Read the model definition and answer for the solid it produces. Units are mm, in the model's axes. Face numbers are marked on the shaded views. A direction names the side the tool comes from. Give positions to 0.01 mm unless a question says otherwise; leave off trailing zeros. Write each loop counter-clockwise with the first axis right and the second up, starting at its lowest first coordinate (ties: lowest second). Pieces come first, ordered by that corner, then holes. Notation, with made-up numbers: M -27,65 L 16,65 A18 ccw 16,86 Z; hole C -37.5,60 d5. An arc over 180 degrees is marked long. Write each question's results on one line, items separated by ' | '. Start each with the question number.
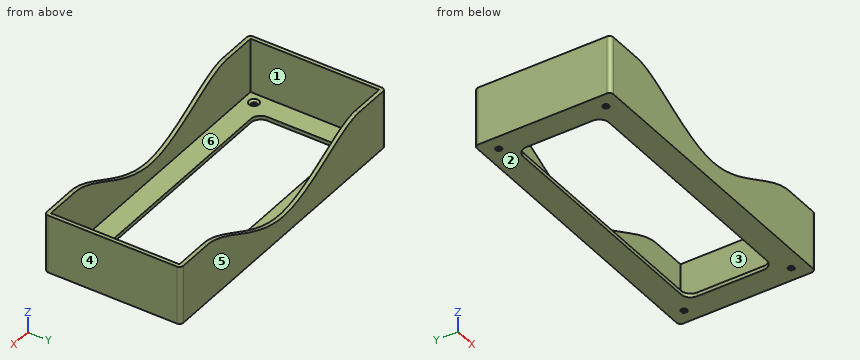
```python
from build123d import *

# Parameters (mm, degrees)
F1_W          = 152
F1_H          = 66
F2_DEPTH      = 30
F1_R          = 1.5875
F3_DEPTH      = 2
F4_SIZE       = 1
F6_DEPTH      = 35
F6_DEPTH_BACK = 35


with BuildPart() as f2:
    # F1 (on Top) → F2 (new body)
    with BuildSketch(Plane.XY):
        with BuildLine():
            ThreePointArc((78, 33), (77.4142135624, 34.4142135624), (76, 35))
            Line((76, 35), (-76, 35))
            ThreePointArc((-76, 35), (-77.4142135624, 34.4142135624), (-78, 33))
            Line((-78, 33), (-78, -33))
            ThreePointArc((-78, -33), (-77.4142135624, -34.4142135624), (-76, -35))
            Line((-76, -35), (76, -35))
            ThreePointArc((76, -35), (77.4142135624, -34.4142135624), (78, -33))
            Line((78, -33), (78, 33))
        make_face()
        Rectangle(F1_W, F1_H, mode=Mode.SUBTRACT)
    extrude(amount=F2_DEPTH)

    # F1 (on Top) → F3 (join)
    with BuildSketch(Plane.XY):
        with BuildLine():
            ThreePointArc((78, 33), (77.4142135624, 34.4142135624), (76, 35))
            Line((76, 35), (-76, 35))
            ThreePointArc((-76, 35), (-77.4142135624, 34.4142135624), (-78, 33))
            Line((-78, 33), (-78, -33))
            ThreePointArc((-78, -33), (-77.4142135624, -34.4142135624), (-76, -35))
            Line((-76, -35), (76, -35))
            ThreePointArc((76, -35), (77.4142135624, -34.4142135624), (78, -33))
            Line((78, -33), (78, 33))
        make_face()
        Rectangle(F1_W, F1_H, mode=Mode.SUBTRACT)
        Rectangle(F1_W, F1_H)
        with Locations((-70.5, -27.5)):
            Circle(F1_R, mode=Mode.SUBTRACT)
        with Locations((70.5, -27.5)):
            Circle(F1_R, mode=Mode.SUBTRACT)
        with Locations((-70.5, 27.5)):
            Circle(F1_R, mode=Mode.SUBTRACT)
        with BuildLine():
            Line((-60, 22), (60, 22))
            ThreePointArc((60, 22), (63.5355339059, 20.5355339059), (65, 17))
            Line((65, 17), (65, -17))
            ThreePointArc((65, -17), (63.5355339059, -20.5355339059), (60, -22))
            Line((60, -22), (-60, -22))
            ThreePointArc((-60, -22), (-63.5355339059, -20.5355339059), (-65, -17))
            Line((-65, -17), (-65, 17))
            ThreePointArc((-65, 17), (-63.5355339059, 20.5355339059), (-60, 22))
        make_face(mode=Mode.SUBTRACT)
        with Locations((70.5, 27.5)):
            Circle(F1_R, mode=Mode.SUBTRACT)
    extrude(amount=F3_DEPTH)

    # F4
    f4_edges = [f2.edges().sort_by_distance(p)[0] for p in [
        (-72.0875, 27.5, 2),
        (68.9125, 27.5, 2),
        (68.9125, -27.5, 2),
        (-72.0875, -27.5, 2),
    ]]
    chamfer(f4_edges, length=F4_SIZE)

    # F5 (on Front) → F6 (cut, two sides)
    with BuildSketch(Plane.XZ) as f6_sk:
        with BuildLine():
            add(Edge.make_bspline(
                [(-58, 30), (-43, 30), (0, -10), (43, 30), (58, 30)],
                knots=[0, 0, 0, 0, 0.5, 1, 1, 1, 1], degree=3))
            Line((58, 30), (-58, 30))
        make_face()
    extrude(amount=-F6_DEPTH, mode=Mode.SUBTRACT)
    extrude(f6_sk.sketch, amount=F6_DEPTH_BACK, mode=Mode.SUBTRACT)


solid = f2.part
```
Item 1: Section B-B, the plane y = 10 is taken. Determine the outline of the cut face in (x, z), then the cut area to 3 significant figures.
Item 2: Straight lines are drawn through the part: line 1 (Y direction, x = -70.5, z = 0.2); line 2 (Y direction, x = -43.5, z = 8); line 3 (X direction, y = -5, z = 17). For each, find the intervals that lie inside material, in ascending order.
Item 3: Determine the mould class of the marked faces 3, 4, 5 and 6 for opening direction X: +X half, -X half, draft (parallel to the pull), parting line (faces both ways), or undercut.
Item 4: Section D-D, the plane y = 27.5 is taken. Determine the outline of the cut face in (x, z), then the cut area to 3 significant figures.
Item 5: Section A-A, the plane x = 70.5 is taken. Determine the outline of the cut face in (y, z).
Item 6: Given P1, Ø3.5, axis at x = 70.5, y = -27.5, coming from the +Z side, flat-ended and moving along its own axis, determine where the tip first touches the part or whether it passes through.
Item 7: Section C-C, the plane z = 6.5 is taken. Determine the outline of the cut face in (x, y), then the cut area to 3 significant figures.
Item 8: For the marked faces 1 and 2, determine the directions among +Z, -Z, +X, -X, +Y, -Y from which every point of the face is accessible in a straight line to the end or side of a thin tool.
Worked out:
1) outline: M -78,0 L -65,0 L -65,2 L -76,2 L -76,30 L -78,30 Z; M 65,0 L 78,0 L 78,30 L 76,30 L 76,2 L 65,2 Z | area: 164 mm²
2) line 1: y = -35 to -29.09, -25.91 to 25.91, 29.09 to 35 | line 2: y = -35 to -33, 33 to 35 | line 3: x = -78 to -76, 76 to 78
3) face 3: undercut | face 4: +X half | face 5: draft | face 6: undercut
4) outline: M -78,0 L -72.09,0 L -72.09,1 L -73.09,2 L -76,2 L -76,30 L -78,30 Z; M -68.91,0 L 68.91,0 L 68.91,1 L 67.91,2 L -67.91,2 L -68.91,1 Z; M 72.09,0 L 78,0 L 78,30 L 76,30 L 76,2 L 73.09,2 L 72.09,1 Z | area: 409 mm²
5) outline: M -35,0 L -29.09,0 L -29.09,1 L -30.09,2 L -33,2 L -33,30 L -35,30 Z; M -25.91,0 L 25.91,0 L 25.91,1 L 24.91,2 L -24.91,2 L -25.91,1 Z; M 29.09,0 L 35,0 L 35,30 L 33,30 L 33,2 L 30.09,2 L 29.09,1 Z
6) P1: stops at z = 1.16
7) outline: M -78,-33 A2 ccw -76,-35 L 76,-35 A2 ccw 78,-33 L 78,33 A2 ccw 76,35 L -76,35 A2 ccw -78,33 Z; hole M -76,-33 L 76,-33 L 76,33 L -76,33 Z | area: 885 mm²
8) face 1: +Z | face 2: -Z, +X, -X, +Y, -Y
